The model under review builds one solid part; all positions refer to its coordinate system, in mm. A direction names the side the tool comes from. Round coordinates to 2 decimals unless told otherwise and drop trailing zeros. Loops run counter-clockwise (first coordinate to the right, second up) from the corner with the lowest first, then second, coordinate; pieces in that order, holes last. Notation, with made-up numbers: M -5.75,71 L 53.25,71 A20 ccw 53.25,80 Z; hole C 28,11 d4. An arc over 180 degrees is marked long. Answer in a Markdown table with one row per item. Add a question column.
from build123d import *

# Parameters (mm, degrees)
SKETCH_6_R           = 6
EXTRUDE_3_DEPTH      = 6
SKETCH_7_R           = 3
EXTRUDE_4_DEPTH      = 12
SKETCH_8_R           = 1.5
CUT_EXTRUDE_22_DEPTH = 12


with BuildPart() as part:
    # 草图5 → 旋转1 (revolve)
    with BuildSketch(Plane.XY):
        with BuildLine():
            Line((0, 0), (0, 18))
            Line((0, 18), (24, 18))
            Line((24, 18), (24, 17.7))
            ThreePointArc((24, 17.7), (24.087867966, 17.912132034), (24.3, 18))
            Line((24.3, 18), (25.5, 18))
            Line((25.5, 18), (25.5, 18.5))
            Line((25.5, 18.5), (48.3, 18.5))
            Line((48.3, 18.5), (48.3, 18))
            Line((48.3, 18), (74, 18))
            Line((74, 18), (74, 6))
            Line((74, 6), (76.7, 6))
            Line((76.7, 6), (76.7, 18))
            Line((76.7, 18), (88.7, 18))
            Line((88.7, 18), (88.7, 0))
            Line((88.7, 0), (0, 0))
        make_face()
    revolve(axis=Axis((-65.679090957, 0, 0), (1, 0, 0)))

    # 草图6 → 凸台-拉伸3 (add)
    with BuildSketch(Plane.ZY):
        with Locations((0, 7)):
            Circle(SKETCH_6_R)
    extrude(amount=EXTRUDE_3_DEPTH)

    # 草图7 → 凸台-拉伸4 (add)
    with BuildSketch(Plane.ZY.offset(6)):
        with Locations((0, 7)):
            Circle(SKETCH_7_R)
    extrude(amount=EXTRUDE_4_DEPTH)

    # 草图8 → 切除-拉伸22 (cut)
    with BuildSketch(Plane.ZY):
        with Locations((15.5, 0)):
            Circle(SKETCH_8_R)
        with Locations((7.75, -13.423393759)):
            Circle(SKETCH_8_R)
        with Locations((-7.75, -13.423393759)):
            Circle(SKETCH_8_R)
        with Locations((-15.5, 0)):
            Circle(SKETCH_8_R)
        with Locations((-7.75, 13.423393759)):
            Circle(SKETCH_8_R)
        with Locations((7.75, 13.423393759)):
            Circle(SKETCH_8_R)
    extrude(amount=-CUT_EXTRUDE_22_DEPTH, mode=Mode.SUBTRACT)


solid = part.part
1. Mouldability with a two-part tool opening along X and no side actions: class faces 4 (the flat face through (88.7, 0, 0)), 5 (the cylindrical face through (37.06, -4.01, -18.06)), 6 (the flat face through (76.7, 0, -8)) as released by +X, released by -X, zero draft, split by the parting line, or undercut.
2. To check wall thickness, follow probe 1 along X at (y, z) = (-14, 2); probe 2 along Z at (x, y) = (4.5, 14); probe 3 along Y at (x, z) = (9, 7). State the ranges of each line that lie inside material, in increasing order.
3. For pin 1 Ø10 at (x, z) = (-4.5, 1) entering from -Y; pin 2 Ø10 at (x, y) = (56, 1) entering from +Z; pin 3 Ø2.5 at (y, z) = (-14, -8.5) entering from -X, all flat-tipped, find the tip position at first contact; note any pin that passes through.
4. Take a section at C-C, the plane x = 15. State the section outline as (y, z) points, and give its area (3 significant figures).
5. Machinability: for faces 1 (the cylindrical face through (61.33, -2.343, 17.847)), 2 (the cylindrical face through (75, -6, 0)), 3 (the flat face through (12, 13, -8)), which of the approach directions +Z, -Z, +X, -X, +Y, -Y give a long, thin tool a straight path to every point of the face, cutting with its end or side? Answer none if there is none.
Check sheet entries:
| question | item | result |
|---|---|---|
| 1 | face 4 | released by +X |
| 1 | face 5 | zero draft |
| 1 | face 6 | undercut |
| 2 | probe 1 | x = 0 to 74, 76.7 to 88.7 |
| 2 | probe 2 | z = -11.31 to -9.13, -6.37 to 6.37, 9.13 to 11.31 |
| 2 | probe 3 | y = -16.58 to -14.72, -12.12 to 12.12, 14.72 to 16.58 |
| 3 | pin 1 | stops at y = -18 |
| 3 | pin 2 | stops at z = 18 |
| 3 | pin 3 | stops at x = 0 |
| 4 | outline | C 0,0 d36 |
| 4 | area | 1,020 mm^2 |
| 5 | face 1 | +X |
| 5 | face 2 | none |
| 5 | face 3 | -X |
